Design review of the part shown in the three views and the two pictorial views. Dimensions are in mm from the part's minimum x, y and z. Round coordinates to 2 decimals unless told otherwise and drop trailing zeros. Write each loop counter-clockwise with the first axis right and the second up, starting at its lowest first coordinate (ties: lowest second). Pieces come first, ordered by that corner, then holes. Notation, with made-up numbers: (28.5, -35) - (62.5, -35) arc R23 cw to (62.5, -21) - close; hole circle Ø9 at (-12, 13.5). An arc over 180 degrees is marked (long way). Use one line per item in the form item = value.
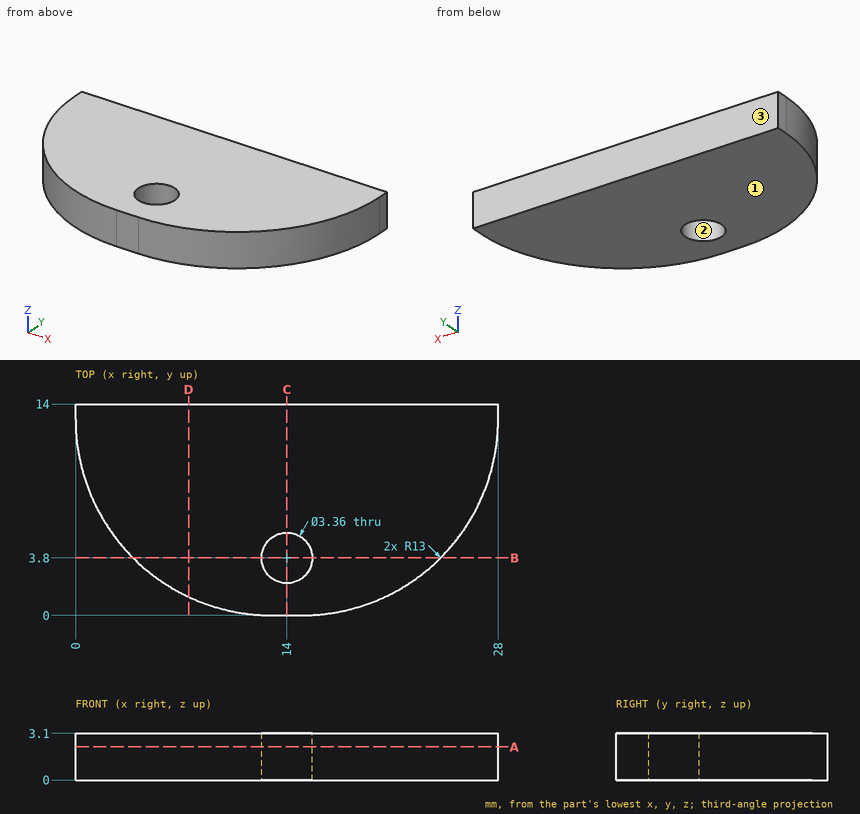
Q1. To check wall thickness, follow line 1 along Y through (x, z) = (14, 1.7); line 2 along Y through (x, z) = (13.5, 0.3); line 3 along X through (y, z) = (6.5, 2.4). State the ranges of each line that lie inside material, in increasing order. Write a range as from..to.
Calculated:
line_1 = 0..2.12, 5.48..14
line_2 = 0..2.2, 5.4..14
line_3 = 1.74..26.26
Q2. Draft analysis for pull direction Y (two halves, no side actions). For the marked faces 1, 2 and 3, state which applies: released by +Y, released by -Y, zero draft, split by the parting line, or undercut.
Calculated:
face_1 = zero draft
face_2 = undercut
face_3 = released by +Y
Q3. We need section C-C on x = 14. Write out the cut boundary in (y, z).
Calculated:
outline = (0, 0) - (2.12, 0) - (2.12, 3.1) - (0, 3.1) - close; (5.48, 0) - (14, 0) - (14, 3.1) - (5.48, 3.1) - close
Q4. For P1, Ø1.5, axis at x = 25, z = 2, coming from the -Y side; P2, Ø1.5, axis at x = 6, z = 1, coming from the -Y side, all flat-tipped, find the tip position at first contact; note any pin that passes through.
Calculated:
P1 = 3.87
P2 = 1.6
Q5. We need section A-A on z = 2.2. Write out the cut boundary in (x, y), then the cut area to 3 significant figures.
Calculated:
outline = (0, 13) arc R13 ccw to (13, 0) - (15, 0) arc R13 ccw to (28, 13) - (28, 14) - (0, 14) - close; hole circle Ø3.36 at (14, 3.8)
area = 311 mm2
Q6. We need section B-B on y = 3.8. Write out the cut boundary in (x, z).
Calculated:
outline = (3.82, 0) - (12.32, 0) - (12.32, 3.1) - (3.82, 3.1) - close; (15.68, 0) - (24.18, 0) - (24.18, 3.1) - (15.68, 3.1) - close
Q7. We need section D-D on x = 7.5. Write out the cut boundary in (y, z).
Calculated:
outline = (1.22, 0) - (14, 0) - (14, 3.1) - (1.22, 3.1) - close
